from build123d import *

# Parameters (mm, degrees)
SKETCH1_W            = 71.3
SKETCH1_H            = 26.8
BOSS_EXTRUDE1_DEPTH  = 0.8
SKETCH2_W            = 71.3
SKETCH2_H            = 26.8
SKETCH2_W_2          = 69.7
SKETCH2_H_2          = 25.2
BOSS_EXTRUDE2_DEPTH  = 7.3
CUT_EXTRUDE1_DEPTH   = 73.91460759
CUT_EXTRUDE4_DEPTH   = 46.193500639
CUT_EXTRUDE5_DEPTH   = 39.937032501
SKETCH13_W           = 2
SKETCH13_H           = 0.8
SKETCH13_W_2         = 1.982692709
SKETCH13_W_3         = 2.017307291
BITIS_DEPTH          = 1.9
SKETCH14_W           = 5
SKETCH14_H           = 0.8
COKOR_DEPTH          = 2
CUT_EXTRUDE6_DEPTH   = 0.5
FILLET1_R            = 0.2
FILLET1_OF_MIRROR1_R = 0.2
CUT_EXTRUDE7_REACH   = 41.931


with BuildPart() as part:
    # Sketch1 → Boss-Extrude1 (new body)
    with BuildSketch(Plane(origin=(0, 0, 0), x_dir=(1, 0, 0), z_dir=(0, 1, 0))):
        Rectangle(SKETCH1_W, SKETCH1_H)
    extrude(amount=BOSS_EXTRUDE1_DEPTH)

    # Sketch2 → Boss-Extrude2 (add)
    with BuildSketch(Plane.XZ):
        Rectangle(SKETCH2_W, SKETCH2_H)
        Rectangle(SKETCH2_W_2, SKETCH2_H_2, mode=Mode.SUBTRACT)
    extrude(amount=BOSS_EXTRUDE2_DEPTH)

    # Sketch5 → Cut-Extrude1 (cut, through all)
    with BuildSketch(Plane.ZY.offset(35.65)):
        with BuildLine():
            Line((-12.4, 0), (-12.6, 0))
            Line((-12.6, 0), (-12.6, -7.3))
            Line((-12.6, -7.3), (12.6, -7.3))
            Line((12.6, -7.3), (12.6, 0))
            Line((12.6, 0), (12.4, 0))
            Line((12.4, 0), (12.4, -3.2))
            Line((12.4, -3.2), (9.6, -3.2))
            Line((9.6, -3.2), (9.6, -2))
            ThreePointArc((9.6, -2), (9.307106781, -1.292893219), (8.6, -1))
            Line((8.6, -1), (-8.6, -1))
            ThreePointArc((-8.6, -1), (-9.307106781, -1.292893219), (-9.6, -2))
            Line((-9.6, -2), (-9.6, -3.2))
            Line((-9.6, -3.2), (-12.4, -3.2))
            Line((-12.4, -3.2), (-12.4, 0))
        make_face()
        with BuildLine():
            Line((13.4, 0.8), (13.4, 0))
            ThreePointArc((13.4, 0), (13.165685425, 0.565685425), (12.6, 0.8))
            Line((12.6, 0.8), (13.4, 0.8))
        make_face()
        with BuildLine():
            Line((-12.6, 0.8), (-13.4, 0.8))
            Line((-13.4, 0.8), (-13.4, 0))
            ThreePointArc((-13.4, 0), (-13.165685425, 0.565685425), (-12.6, 0.8))
        make_face()
    extrude(amount=-CUT_EXTRUDE1_DEPTH, mode=Mode.SUBTRACT)

    # Sketch9 → Cut-Extrude4 (cut, through all)
    with BuildSketch(Plane.XY.offset(13.4)):
        with BuildLine():
            ThreePointArc((-34.85, 0.8), (-35.415685425, 0.565685425), (-35.65, 0))
            Line((-35.65, 0), (-35.65, 0.8))
            Line((-35.65, 0.8), (-34.85, 0.8))
        make_face()
        Polygon((-34.65, 0), (-34.85, 0), (-34.85, -3.2), (-35.65, -3.2), (-35.65, -7.3), (-34.65, -7.3), align=None)
        Polygon((34.85, 0), (34.65, 0), (34.65, -7.3), (35.65, -7.3), (35.65, -3.2), (34.85, -3.2), align=None)
        with BuildLine():
            Line((35.65, 0.8), (35.65, 0))
            ThreePointArc((35.65, 0), (35.415685425, 0.565685425), (34.85, 0.8))
            Line((34.85, 0.8), (35.65, 0.8))
        make_face()
    extrude(amount=-CUT_EXTRUDE4_DEPTH, mode=Mode.SUBTRACT)

    # Sketch10 → Cut-Extrude5 (cut, through all)
    with BuildSketch(Plane(origin=(0, 0.8, 0), x_dir=(1, 0, 0), z_dir=(0, 1, 0))):
        Polygon((-34.65, -12.6), (-34.65, -13.4), (-35.65, -13.4), (-35.65, -12.4), (-34.85, -12.4), align=None)
        Polygon((35.65, -13.4), (34.65, -13.4), (34.65, -12.6), (34.85, -12.4), (35.65, -12.4), align=None)
        Polygon((34.65, 12.6), (34.65, 13.4), (35.65, 13.4), (35.65, 12.4), (34.85, 12.4), align=None)
        Polygon((-35.65, 13.4), (-34.65, 13.4), (-34.65, 12.6), (-34.85, 12.4), (-35.65, 12.4), align=None)
    extrude(amount=-CUT_EXTRUDE5_DEPTH, mode=Mode.SUBTRACT)

    # Sketch13 → Bitis (add)
    with BuildSketch(Plane.XZ.offset(7.3)):
        with Locations((31.479809087, 13)):
            Rectangle(SKETCH13_W, SKETCH13_H)
        with Locations((31.302010091, -13)):
            Rectangle(SKETCH13_W, SKETCH13_H)
        with Locations((1.258653645, -13)):
            Rectangle(SKETCH13_W_2, SKETCH13_H)
        with Locations((-28.741346355, 13)):
            Rectangle(SKETCH13_W_3, SKETCH13_H)
        with Locations((1.258653645, 13)):
            Rectangle(SKETCH13_W_2, SKETCH13_H)
        with Locations((-28.741346355, -13)):
            Rectangle(SKETCH13_W_3, SKETCH13_H)
    extrude(amount=BITIS_DEPTH)

    # Sketch14 → Cokor (add)
    with BuildSketch(Plane.XZ.offset(9.2)):
        with Locations((-27.25, 13)):
            Rectangle(SKETCH14_W, SKETCH14_H)
        with Locations((2.767307291, -13)):
            Rectangle(SKETCH14_W, SKETCH14_H)
        with Locations((-27.25, -13)):
            Rectangle(SKETCH14_W, SKETCH14_H)
        with Locations((2.767307291, 13)):
            Rectangle(SKETCH14_W, SKETCH14_H)
        with Locations((32.979809087, 13)):
            Rectangle(SKETCH14_W, SKETCH14_H)
        with Locations((32.802010091, -13)):
            Rectangle(SKETCH14_W, SKETCH14_H)
    extrude(amount=COKOR_DEPTH)

    # Sketch15 → Cut-Extrude6 (cut)
    with BuildSketch(Plane(origin=(0, 0.8, 0), x_dir=(1, 0, 0), z_dir=(0, 1, 0))):
        with BuildLine():
            Line((-32.5, -10.588064309), (32.5, -10.588064309))
            ThreePointArc((32.5, -10.588064309), (33, -11.088064309), (32.5, -11.588064309))
            Line((32.5, -11.588064309), (-32.5, -11.588064309))
            ThreePointArc((-32.5, -11.588064309), (-33, -11.088064309), (-32.5, -10.588064309))
        make_face()
    cut_extrude6 = extrude(amount=-CUT_EXTRUDE6_DEPTH, mode=Mode.SUBTRACT)

    # Fillet1
    fillet1_edges = [part.edges().sort_by_distance(p)[0] for p in [
        (-33, 0.3, 11.088064309),
        (0, 0.3, 10.588064309),
        (33, 0.3, 11.088064309),
        (0, 0.3, 11.588064309),
        (-33, 0.8, 11.088064309),
        (0, 0.8, 11.588064309),
        (33, 0.8, 11.088064309),
        (0, 0.8, 10.588064309),
    ]]
    fillet(fillet1_edges, radius=FILLET1_R)

    # Mirror1: Cut-Extrude6 across plane
    add(cut_extrude6.mirror(Plane.XY), mode=Mode.SUBTRACT)

    # Fillet1 of Mirror1
    fillet1_of_mirror1_edges = [part.edges().sort_by_distance(p)[0] for p in [
        (-33, 0.3, -11.088064309),
        (0, 0.3, -10.588064309),
        (33, 0.3, -11.088064309),
        (0, 0.3, -11.588064309),
        (-33, 0.8, -11.088064309),
        (0, 0.8, -11.588064309),
        (33, 0.8, -11.088064309),
        (0, 0.8, -10.588064309),
    ]]
    fillet(fillet1_of_mirror1_edges, radius=FILLET1_OF_MIRROR1_R)

    # Sketch19 → Cut-Extrude7 (cut, up to next)
    with BuildSketch(Plane(origin=(0, 0.8, 0), x_dir=(1, 0, 0), z_dir=(0, 1, 0)), mode=Mode.PRIVATE) as cut_extrude7_sk1:
        with BuildLine():
            Line((-31.280382084, -6.979906863), (31.219617916, -6.979906863))
            ThreePointArc((31.219617916, -6.979906863), (31.926724698, -6.687013644), (32.219617916, -5.979906863))
            Line((32.219617916, -5.979906863), (32.219617916, 5.820093137))
            ThreePointArc((32.219617916, 5.820093137), (31.926724698, 6.527199918), (31.219617916, 6.820093137))
            Line((31.219617916, 6.820093137), (-31.280382084, 6.820093137))
            ThreePointArc((-31.280382084, 6.820093137), (-31.987488865, 6.527199918), (-32.280382084, 5.820093137))
            Line((-32.280382084, 5.820093137), (-32.280382084, -5.979906863))
            ThreePointArc((-32.280382084, -5.979906863), (-31.987488865, -6.687013644), (-31.280382084, -6.979906863))
        make_face()
    cut_extrude7_tool1 = extrude(cut_extrude7_sk1.sketch, amount=-CUT_EXTRUDE7_REACH, mode=Mode.PRIVATE) & part.part
    add(cut_extrude7_tool1.solids().sort_by_distance((-0.030382, 0.8, 0.079907))[0], mode=Mode.SUBTRACT)


solid = part.part
Read the model definition and answer for the solid it produces. Units are mm, in the model's axes. A direction names the side the tool comes from. Give positions to 0.01 mm unless a question says otherwise; leave off trailing zeros. Write each loop counter-clockwise with the first axis right and the second up, starting at its lowest first coordinate (ties: lowest second). Pieces come first, ordered by that corner, then holes. Notation, with made-up numbers: (35, 18) - (40, 18) arc R14 cw to (40, 41) - close; hole circle Ø6 at (49.5, 57.25). An arc over 180 degrees is marked (long way). Return JSON: item names as keys, results as strings.
Q1. A cutting plane is placed at C-C, the plane y = -5.25. Determine the outline of the cut face in (x, z).
Reply:
{"outline": "(-34.65, -13.4) - (34.65, -13.4) - (34.65, -12.6) - (-34.65, -12.6) - close; (-34.65, 12.6) - (34.65, 12.6) - (34.65, 13.4) - (-34.65, 13.4) - close"}
Q2. Given P1, Ø2, axis at x = -28.5, z = -8, coming from the -Y side; P2, Ø0.6, axis at y = -9, z = 13, coming from the -X side; P3, Ø3.5, axis at y = -2, z = -1, coming from the +X side; P4, Ø0.9, axis at x = 35, z = -11, coming from the -Y side, each flat-ended and moving along its own axis, determine where each tip first touches the part or whether it passes through.
Reply:
{"P1": "y = 0", "P2": "x = -29.75", "P3": "x = 35.65", "P4": "y = -3.2"}
Q3. For faces 5 (the face through (0, -4, -13.4)), 6 (the face through (0, 0, 9)), 7 (the face through (-34.85, -0.5, -0.2)), determine the directions among +Z, -Z, +X, -X, +Y, -Y from which every point of the face is accessible in a straight line to the end or side of a thin tool.
Reply:
{"face 5": "-Z, +X, -X, +Y, -Y", "face 6": "-Y", "face 7": "+Z, -Z, -Y"}
Q4. A cutting plane is placed at A-A, the plane z = 1. Determine the outline of the cut face in (x, y).
Reply:
{"outline": "(-35.65, -1) - (-34.85, -1) - (-34.85, 0) - (-32.28, 0) - (-32.28, 0.8) - (-34.85, 0.8) arc R0.8 ccw to (-35.65, 0) - close; (32.22, 0) - (34.85, 0) - (34.85, -1) - (35.65, -1) - (35.65, 0) arc R0.8 ccw to (34.85, 0.8) - (32.22, 0.8) - close"}
Q5. Consider line 1 along Z through (x, y) = (14, -3.75); line 2 along X through (y, z) = (-0.75, -8.25); line 3 along Y through (x, z) = (-12.5, 11.75). Determine where each line is inside the solid, lowest interval first. Write a range as [from, to].
Reply:
{"line 1": "[-13.4, -12.6], [12.6, 13.4]", "line 2": "[-35.65, -34.85], [34.85, 35.65]", "line 3": "[0, 0.8]"}
Q6. For a pull along Z with two mould halves and no side action, classify faces 1 (the face through (0, -4, -12.6)), 2 (the face through (34.85, -0.5, -0.2)), 3 (the face through (0, -4, 13.4)), 4 (the face through (0, -4, 12.6)) as released by +Z, released by -Z, zero draft, split by the parting line, or undercut.
Reply:
{"face 1": "undercut", "face 2": "zero draft", "face 3": "released by +Z", "face 4": "undercut"}
